The model under review builds one solid part; all positions refer to its coordinate system, in mm. A direction names the side the tool comes from. Round coordinates to 2 decimals unless told otherwise and drop trailing zeros. Order: outer loops, then holes, each group sorted by start corner. A loop starts at its lowest first (then second) coordinate and runs counter-clockwise, first axis right, second up.
Autodesk Inventor part; units mm, degrees
ref_plane "YZ Plane" through (0, 0, 0) normal (1, 0, 0) x (0, 1, 0)
ref_plane "XZ Plane" through (0, 0, 0) normal (0, 1, 0) x (-1, 0, 0)
ref_plane "XY Plane" through (0, 0, 0) normal (0, 0, 1) x (1, 0, 0)
sketch "Sketch12" plane through (0, 0, 0) normal (0, 1, 0) x (-1, 0, 0)
  line L0 (0, 0) -> (0, -102.5) construction
  line L1 (0, 0) -> (0, 102.5) construction
  line L2 (0, 102.5) -> (125, 102.5) construction
  line L3 (125, 102.5) -> (125, -102.5) construction
  line L4 (125, -102.5) -> (0, -102.5) construction
  line L5 (0, -102.5) -> (0, 102.5) construction
  line L6 (0, 102.5) -> (45, 102.5) construction
  line L7 (45, 102.5) -> (45, -102.5) construction
  line L8 (45, -102.5) -> (0, -102.5) construction
  line L9 (0, -102.5) -> (0, 102.5) construction
  line L10 (125, 0) -> (125, -217.5) construction
  line L11 (125, 0) -> (125, 217.5) construction
  line L12 (125, 217.5) -> (72.0108, 217.5) construction
  line L13 (45, 217.5) -> (45, 102.5) construction
  line L14 (125, -217.5) -> (72.0108, -217.5) construction
  line L15 (45, -217.5) -> (45, -102.5) construction
  arc A0 (34.5307, 191.4729) -> (34.5307, -191.4729) centre (548.125, 0) ccw construction
  arc A1 (34.5307, -191.4729) -> (72.0108, -217.5) centre (72.0108, -177.5) ccw construction
  arc A2 (72.0108, 217.5) -> (34.5307, 191.4729) centre (72.0108, 177.5) ccw construction
  line L16 (125, -102.5) -> (125, 102.5)
  line L17 (125, 102.5) -> (9.6691, 102.5)
  line L18 (125, -102.5) -> (9.6691, -102.5)
  arc A3 (9.6691, 102.5) -> (9.6691, -102.5) centre (548.125, 0) ccw construction
  line L19 (9.6691, 102.5) -> (9.6691, -102.5)
  dimension "d698" = 102.5
  dimension "d699" = 102.5
  dimension "d700" = 125
  dimension "d701" = 45
  dimension "d702" = 217.5
  dimension "d703" = 217.5
  dimension "d704" = 40
extrude "Extrusion12" add sketch "Sketch12" along normal blind 115
sketch "Sketch84" plane through (-125, 0, -102.5) normal (-1, 0, 0) x (0, 0, 1)
  line L0 (30.5, 113.5) -> (174.5, 113.5)
  line L1 (182.5, 105.5) -> (182.5, 9.5)
  line L2 (174.5, 1.5) -> (30.5, 1.5)
  line L3 (22.5, 9.5) -> (22.5, 105.5)
  line L4 (205, 0) -> (205, 115)
  line L5 (0, 0) -> (0, 115)
  line L6 (0, 115) -> (205, 115)
  line L7 (0, 0) -> (205, 0)
  arc A0 (30.5, 113.5) -> (22.5, 105.5) centre (30.5, 105.5) ccw
  arc A1 (182.5, 105.5) -> (174.5, 113.5) centre (174.5, 105.5) ccw
  arc A2 (174.5, 1.5) -> (182.5, 9.5) centre (174.5, 9.5) ccw
  arc A3 (22.5, 9.5) -> (30.5, 1.5) centre (30.5, 9.5) ccw
  point P0 (102.5, 0)
  dimension "d705" = 22.5
  dimension "d706" = 22.5
  dimension "d707" = 1.5
  dimension "d708" = 1.5
  dimension "d709" = 8
extrude "Extrusion69" cut sketch "Sketch84" against normal blind 102 contours L0 A1 L1 A2 L2 A3 L3 A0
sketch "Sketch85" plane through (-125, 0, -102.5) normal (-1, 0, 0) x (0, 0, 1)
  line L0 (205, 0) -> (205, 97)
  line L1 (205, 25) -> (205, 40)
  line L2 (205, 32.5) -> (185, 32.5) construction
  line L3 (185, 32.5) -> (185, 47.5)
  line L4 (185, 32.5) -> (185, 17.5)
  line L5 (205, 40) -> (195, 40)
  line L6 (195, 40) -> (185, 47.5)
  line L7 (205, 25) -> (195, 25)
  line L8 (195, 25) -> (185, 17.5)
  line L9 (0, 0) -> (205, 0)
  line L10 (205, 75) -> (205, 90)
  line L11 (205, 82.5) -> (185, 82.5) construction
  line L12 (185, 82.5) -> (185, 97.5)
  line L13 (185, 82.5) -> (185, 67.5)
  line L14 (205, 75) -> (195, 75)
  line L15 (195, 75) -> (185, 67.5)
  line L16 (205, 90) -> (195, 90)
  line L17 (195, 90) -> (185, 97.5)
  line L18 (0, 115) -> (205, 115)
  line L19 (0, 0) -> (0, 115)
  line L20 (0, 25) -> (10, 25)
  line L21 (0, 25) -> (10, 25) construction
  line L22 (0, 25) -> (0, 40)
  line L23 (10, 40) -> (0, 40)
  line L24 (0, 32.5) -> (20, 32.5) construction
  line L25 (20, 32.5) -> (20, 47.5)
  line L26 (20, 47.5) -> (10, 40)
  line L27 (20, 32.5) -> (20, 17.5)
  line L28 (20, 17.5) -> (10, 25)
  line L29 (0, 90) -> (10, 90)
  line L30 (0, 90) -> (0, 75)
  line L31 (10, 75) -> (0, 75)
  line L32 (0, 82.5) -> (20, 82.5) construction
  line L33 (20, 82.5) -> (20, 97.5)
  line L34 (20, 97.5) -> (10, 90)
  line L35 (20, 82.5) -> (20, 67.5)
  line L36 (20, 67.5) -> (10, 75)
  point P0 (102.5, 0)
  dimension "d712" = 15
  dimension "d713" = 20
  dimension "d714" = 15
  dimension "d715" = 15
  dimension "d717" = 10
  dimension "d718" = 25
  dimension "d719" = 15
  dimension "d720" = 20
  dimension "d721" = 15
  dimension "d722" = 15
  dimension "d723" = 10
  dimension "d728" = 25
  dimension "d732" = 10
  dimension "d734" = 20
  dimension "d735" = 15
  dimension "d736" = 15
extrude "Extrusion70" cut sketch "Sketch85" against normal blind 100
sketch "Sketch86" plane through (-9.6691, 0, 102.5) normal (1, 0, 0) x (0, 0, -1)
  line L0 (0, 90) -> (0, 115) construction
  line L1 (0, 0) -> (205, 0) construction
  line L2 (0, 115) -> (205, 0) construction
  line L3 (0, 115) -> (205, 115) construction
  line L4 (205, 115) -> (0, 0) construction
  line L5 (191.5, 1.5) -> (13.5, 1.5)
  line L6 (5.5, 9.5) -> (5.5, 105.5)
  line L7 (13.5, 113.5) -> (191.5, 113.5)
  line L8 (199.5, 105.5) -> (199.5, 9.5)
  line L9 (199.5, 1.5) -> (5.5, 113.5) construction
  line L10 (5.5, 1.5) -> (199.5, 113.5) construction
  arc A0 (13.5, 113.5) -> (5.5, 105.5) centre (13.5, 105.5) ccw
  arc A1 (199.5, 105.5) -> (191.5, 113.5) centre (191.5, 105.5) ccw
  arc A2 (191.5, 1.5) -> (199.5, 9.5) centre (191.5, 9.5) ccw
  arc A3 (5.5, 9.5) -> (13.5, 1.5) centre (13.5, 9.5) ccw
  point P0 (102.5, 0)
  point P1 (102.5, 57.5)
  dimension "d738" = 194
  dimension "d739" = 112
  dimension "d740" = 8
extrude "Extrusion71" cut sketch "Sketch86" against normal blind 8.9
sketch "Sketch90" plane through (-18.5691, 0, 102.5) normal (1, 0, 0) x (0, 0, -1)
  circle A0 centre (41.2486, 90.9267) radius 1.75
  circle A1 centre (167.2486, 25.4267) radius 1.75
  circle A2 centre (41.2486, 25.4267) radius 1.75
  circle A3 centre (167.2486, 90.9267) radius 1.75
  line L0 (198.9986, 106.9003) -> (198.9986, 7.9003)
  line L1 (190.9986, 1.9267) -> (13.9986, 1.9267) construction
  line L2 (5.9986, 9.9267) -> (5.9986, 104.9267) construction
  line L3 (13.9986, 112.9267) -> (190.9986, 112.9267) construction
  line L4 (198.9986, 104.9267) -> (198.9986, 9.9267) construction
  arc A4 (13.9986, 112.9267) -> (5.9986, 104.9267) centre (13.9986, 104.9267) ccw
  arc A5 (198.9986, 104.9267) -> (190.9986, 112.9267) centre (190.9986, 104.9267) ccw
  arc A6 (190.9986, 1.9267) -> (198.9986, 9.9267) centre (190.9986, 9.9267) ccw
  arc A7 (5.9986, 9.9267) -> (13.9986, 1.9267) centre (13.9986, 9.9267) ccw
  line L5 (21.3986, 106.3267) -> (186.7486, 106.3267) construction
  line L6 (186.7486, 106.3267) -> (186.7486, 5.5767) construction
  line L7 (186.7486, 5.5767) -> (21.3986, 5.5767) construction
  line L8 (21.3986, 5.5767) -> (21.3986, 106.3267) construction
  line L9 (33.7486, 94.9267) -> (48.7486, 94.9267) construction
  line L10 (48.7486, 94.9267) -> (48.7486, 86.9267) construction
  line L11 (48.7486, 86.9267) -> (33.7486, 86.9267) construction
  line L12 (33.7486, 86.9267) -> (33.7486, 94.9267) construction
  line L13 (33.7486, 94.9267) -> (48.7486, 86.9267) construction
  line L14 (48.7486, 94.9267) -> (33.7486, 86.9267) construction
  line L15 (33.7486, 29.4267) -> (48.7486, 29.4267) construction
  line L16 (48.7486, 29.4267) -> (48.7486, 21.4267) construction
  line L17 (48.7486, 21.4267) -> (33.7486, 21.4267) construction
  line L18 (33.7486, 21.4267) -> (33.7486, 29.4267) construction
  line L19 (33.7486, 29.4267) -> (48.7486, 21.4267) construction
  line L20 (48.7486, 29.4267) -> (33.7486, 21.4267) construction
  line L21 (159.7486, 29.4267) -> (174.7486, 29.4267) construction
  line L22 (174.7486, 29.4267) -> (174.7486, 21.4267) construction
  line L23 (174.7486, 21.4267) -> (159.7486, 21.4267) construction
  line L24 (159.7486, 21.4267) -> (159.7486, 29.4267) construction
  line L25 (159.7486, 29.4267) -> (174.7486, 21.4267) construction
  line L26 (174.7486, 29.4267) -> (159.7486, 21.4267) construction
  line L27 (159.7486, 94.9267) -> (174.7486, 94.9267) construction
  line L28 (174.7486, 94.9267) -> (174.7486, 86.9267) construction
  line L29 (174.7486, 86.9267) -> (159.7486, 86.9267) construction
  line L30 (159.7486, 86.9267) -> (159.7486, 88.953) construction
  line L31 (159.7486, 94.9267) -> (174.7486, 86.9267) construction
  line L32 (174.7486, 94.9267) -> (159.7486, 86.9267) construction
  line L33 (159.7486, 94.9267) -> (159.7486, 84.9003) construction
  line L34 (0, 90) -> (0, 115) construction
  line L35 (205, 0) -> (205, 25) construction
  line L36 (0, 115) -> (205, 0) construction
  line L37 (205, 0) -> (205, 115) construction
  line L38 (0, 0) -> (0, 115) construction
  line L39 (0, 0) -> (205, 115) construction
  line L40 (182.5, 9.5) -> (182.5, 105.5)
  line L41 (13.5, 113.5) -> (191.5, 113.5)
  line L42 (191.5, 1.5) -> (13.5, 1.5)
  line L43 (5.5, 9.5) -> (5.5, 105.5)
  line L44 (199.5, 105.5) -> (199.5, 9.5)
  line L45 (182.5, 80.9267) -> (165.2486, 80.9267)
  line L46 (13.5, 113.5) -> (191.5, 113.5)
  arc A8 (182.5, 105.5) -> (174.5, 113.5) centre (174.5, 105.5) ccw
  line L47 (174.5, 113.5) -> (30.5, 113.5) construction
  line L48 (174.5, 113.5) -> (30.5, 113.5) construction
  line L49 (157.2486, 88.9267) -> (157.2486, 113.5)
  arc A9 (157.2486, 88.9267) -> (165.2486, 80.9267) centre (165.2486, 88.9267) ccw
  line L50 (157.2486, 113.5) -> (174.5, 113.5)
  line L51 (182.5, 80.9267) -> (182.5, 105.5)
  arc A10 (182.5, 105.5) -> (174.5, 113.5) centre (174.5, 105.5) ccw
  line L52 (154.7486, 5.5767) -> (154.7486, 27.4267)
  line L53 (162.7486, 35.4267) -> (182.5, 35.4267)
  arc A11 (174.5, 1.5) -> (182.5, 9.5) centre (174.5, 9.5) ccw
  line L54 (182.5, 9.5) -> (182.5, 35.4267)
  line L55 (174.5, 1.5) -> (154.7486, 1.5)
  arc A12 (174.5, 1.5) -> (182.5, 9.5) centre (174.5, 9.5) ccw
  arc A13 (162.7486, 35.4267) -> (154.7486, 27.4267) centre (162.7486, 27.4267) ccw
  line L56 (48.7486, 1.5) -> (48.7486, 27.4267)
  line L57 (40.7486, 35.4267) -> (22.5, 35.4267)
  line L58 (22.5, 105.5) -> (22.5, 9.5)
  line L59 (22.5, 9.5) -> (22.5, 35.4267)
  line L60 (30.5, 1.5) -> (48.7486, 1.5)
  arc A14 (22.5, 9.5) -> (30.5, 1.5) centre (30.5, 9.5) ccw
  arc A15 (22.5, 9.5) -> (30.5, 1.5) centre (30.5, 9.5) ccw
  arc A16 (48.7486, 27.4267) -> (40.7486, 35.4267) centre (40.7486, 27.4267) ccw
  line L61 (51.2486, 113.5) -> (51.2486, 88.9267)
  line L62 (43.2486, 80.9267) -> (22.5, 80.9267)
  line L63 (22.5, 80.9267) -> (22.5, 105.5)
  line L64 (51.2486, 113.5) -> (30.5, 113.5)
  arc A17 (30.5, 113.5) -> (22.5, 105.5) centre (30.5, 105.5) ccw
  arc A18 (30.5, 113.5) -> (22.5, 105.5) centre (30.5, 105.5) ccw
  arc A19 (43.2486, 80.9267) -> (51.2486, 88.9267) centre (43.2486, 88.9267) ccw
  line L65 (22.5, 80.9267) -> (22.5, 35.4267)
  line L66 (22.5, 105.5) -> (22.5, 9.5)
  line L67 (51.2486, 113.5) -> (157.2486, 113.5)
  line L68 (182.5, 80.9267) -> (182.5, 35.4267)
  line L69 (154.7486, 5.5767) -> (154.7486, 1.5)
  line L70 (0, 0) -> (205, 0)
  line L71 (48.7486, 1.5) -> (48.7486, 1.9267)
  line L72 (154.7486, 1.5) -> (154.7486, 1.9267)
  line L73 (48.7486, 1.5) -> (154.7486, 1.5)
  line L74 (30.5, 1.5) -> (174.5, 1.5)
  point P0 (102.5, 0)
  point P1 (5.9986, 112.9267)
  point P2 (5.9986, 1.9267)
  point P3 (198.9986, 112.9267)
  point P4 (159.7486, 25.4267)
  point P5 (102.4986, 57.5003)
  point P6 (51.2486, 11.5)
  point P7 (179.5, 80.9267)
  point P8 (157.2486, 103.5)
  point P9 (48.7486, 1.5)
  point P10 (154.7486, 1.5)
  dimension "d840" = 3.5
  dimension "d841" = 3.5
  dimension "d842" = 3.5
  dimension "d843" = 3.5
  dimension "d844" = 193
  dimension "d845" = 111
  dimension "d846" = 8
  dimension "d847" = 8
  dimension "d848" = 165.35
  dimension "d849" = 100.75
  dimension "d850" = 3.65
  dimension "d851" = 15.4
  dimension "d852" = 15.4
  dimension "d853" = 19.85
  dimension "d854" = 19.85
  dimension "d855" = 15
  dimension "d856" = 8
  dimension "d857" = 15
  dimension "d858" = 15
  dimension "d859" = 8
  dimension "d860" = 19.5
  dimension "d861" = 19.85
  dimension "d862" = 19.5
  dimension "d863" = 19.85
  dimension "d864" = 12.25
  dimension "d865" = 0
  dimension "d868" = 15.4
  dimension "d869" = 6.6
  dimension "d870" = 12.25
  dimension "d892" = 8
  dimension "d893" = 8
  dimension "d894" = 8
  dimension "d895" = 8
  dimension "d902" = 10
  dimension "d903" = 10
  dimension "d904" = 10
  dimension "d905" = 10
extrude "Extrusion74" cut sketch "Sketch90" against normal blind 10 contours A0 | A1 | A2 | A3 | L53 A13 L52 L69 L42 L56 A16 L57 L58 L62 A19 L61 L41 L49 A9 L45 L40
sketch "Sketch91" plane through (-23, 0, -102.5) normal (-1, 0, 0) x (0, 0, 1)
  circle A0 centre (37.7514, 90.9267) radius 1.75
  circle A1 centre (37.7514, 90.9267) radius 5
  circle A2 centre (163.7514, 90.9267) radius 1.75
  circle A3 centre (163.7514, 90.9267) radius 5
  circle A4 centre (163.7514, 25.4267) radius 1.75
  circle A5 centre (163.7514, 25.4267) radius 5
  circle A6 centre (37.7514, 25.4267) radius 1.75
  circle A7 centre (37.7514, 25.4267) radius 5
  point P0 (102.5, 0)
  dimension "d896" = 10
  dimension "d897" = 10
  dimension "d898" = 10
  dimension "d899" = 10
extrude "Extrusion75" cut sketch "Sketch91" against normal blind 2
properties part number "center_fp13"
(1) Insertion check: pin 1 (5 mm diameter, centred on y = 26, z = -66.5, fed in from -X); pin 2 (8 mm diameter, centred on y = 90.93, z = -64.75, fed in from +X); pin 3 (23 mm diameter, centred on y = 93, z = 65, fed in from -X). Each pin has a flat end and moves straight along its axis. Give the tip position at first contact, or say it passes through.
Data:
pin 1: stops at x = -21
pin 2: stops at x = -18.57
pin 3: stops at x = -23
(2) For faces 1 (the cylindrical face through (-20.75, 33.02, 56.03)), 2 (the flat face through (-75.7, 71.3, 87.57)), 3 (the flat face through (-76, 40, -97)), list the 3-axis set-ups (+Z, -Z, +X, -X, +Y, -Y) from which the entire face can be reached by the end or side of a thin tool; tool diameter is ignored.
Data:
face 1: +X, -X
face 2: -X
face 3: -Z, -X
(3) Consider section B-B (z = -45). Write out the cut boundary in (x, y), and give its area (3 significant figures).
Data:
outline: (-125, 0) - (-9.67, 0) - (-9.67, 1.5) - (-125, 1.5) - close; (-125, 113.5) - (-9.67, 113.5) - (-9.67, 115) - (-125, 115) - close
area: 346 mm2
(4) Consider section D-D (z = 74.5). Write out the cut boundary in (x, y).
Data:
outline: (-125, 0) - (-9.67, 0) - (-9.67, 1.5) - (-18.57, 1.5) - (-18.57, 35.43) - (-23, 35.43) - (-23, 1.9) - (-125, 1.9) - close; (-125, 113.1) - (-23, 113.1) - (-23, 80.93) - (-18.57, 80.93) - (-18.57, 113.5) - (-9.67, 113.5) - (-9.67, 115) - (-125, 115) - close
(5) Consider section C-C (y = 52.5). Write out the cut boundary in (x, z), and give its area (3 significant figures).
Data:
outline: (-125, -102.5) - (-9.67, -102.5) - (-9.67, -97) - (-18.57, -97) - (-18.57, -80) - (-125, -80) - close; (-125, 80) - (-18.57, 80) - (-18.57, 97) - (-9.67, 97) - (-9.67, 102.5) - (-125, 102.5) - close
area: 4,890 mm2
(6) To check wall thickness, follow probe 1 along Z at (x, y) = (-48.5, 88); probe 2 along Y at (x, z) = (-99, -14); probe 3 along Z at (x, y) = (-59, 50). State the ranges of each line that lie inside material, in increasing order.
Data:
probe 1: z = -82.5 to -80, 80 to 82.5
probe 2: y = 0 to 1.5, 113.5 to 115
probe 3: z = -102.5 to -80, 80 to 102.5
(7) Consider section A-A (y = 78.5). Write out the cut boundary in (x, z).
Data:
outline: (-125, -82.5) - (-25, -82.5) - (-25, -102.5) - (-9.67, -102.5) - (-9.67, -97) - (-18.57, -97) - (-18.57, -80) - (-125, -80) - close; (-125, 80) - (-18.57, 80) - (-18.57, 97) - (-9.67, 97) - (-9.67, 102.5) - (-25, 102.5) - (-25, 82.5) - (-125, 82.5) - close
(8) Draft analysis for pull direction Z (two halves, no side actions). For faces 4 (the cylindrical face through (-22.014, 86.046, 60.167)), 5 (the flat face through (-76, 25, -98)), 6 (the flat face through (-68, 57, 102.5)), state which applies: pulls with the +Z half, pulls with the -Z half, needs draft (parallel to the pull), parting line crosses it, or undercut.
Data:
face 4: undercut
face 5: needs draft
face 6: pulls with the +Z half
